Source: CAD feature listing. Evaluate the final solid. Frame: model axes, mm. Coordinates: 2 decimals unless noted, no trailing zeros. Order: outer loops, then holes, each group sorted by start corner. A loop starts at its lowest first (then second) coordinate and runs counter-clockwise, first axis right, second up.
Autodesk Inventor part; units mm, degrees
ref_plane "YZ Plane" through (0, 0, 0) normal (1, 0, 0) x (0, 1, 0)
ref_plane "XZ Plane" through (0, 0, 0) normal (0, 1, 0) x (-1, 0, 0)
ref_plane "XY Plane" through (0, 0, 0) normal (0, 0, 1) x (1, 0, 0)
sketch "Sketch1" plane through (0, 0, 0) normal (0, 0, 1) x (1, 0, 0)
  line L0 (0, 0) -> (127, 0)
  line L1 (127, 0) -> (127, 88.9)
  line L2 (127, 88.9) -> (0, 88.9)
  line L3 (0, 88.9) -> (0, 0)
  circle A0 centre (10.16, 78.74) radius 3.0988
  circle A1 centre (10.16, 44.45) radius 3.0988
  circle A2 centre (10.16, 10.16) radius 3.0988
  circle A3 centre (45.72, 10.16) radius 3.0988
  circle A4 centre (116.84, 10.16) radius 3.0988
  circle A5 centre (116.84, 44.45) radius 3.0988
  circle A6 centre (116.84, 78.74) radius 3.0988
  circle A7 centre (45.72, 78.74) radius 3.0988
  line L4 (25.4, 25.4) -> (101.6, 25.4)
  line L5 (101.6, 25.4) -> (101.6, 63.5)
  line L6 (101.6, 63.5) -> (25.4, 63.5)
  line L7 (25.4, 63.5) -> (25.4, 25.4)
  line L8 (25.4, 25.4) -> (101.6, 63.5) construction
  line L9 (101.6, 25.4) -> (25.4, 63.5) construction
  circle A8 centre (81.28, 10.16) radius 3.0988
  circle A9 centre (81.28, 78.74) radius 3.0988
  point P0 (63.5, 44.45)
  dimension "d0" = 127
  dimension "d1" = 88.9
  dimension "d3" = 6.1976
  dimension "d4" = 10.16
  dimension "d5" = 10.16
  dimension "d6" = 10.16
  dimension "d7" = 10.16
  dimension "d8" = 44.45
  dimension "d10" = 10.16
  dimension "d11" = 10.16
  dimension "d12" = 10.16
  dimension "d13" = 10.16
  dimension "d14" = 44.45
  dimension "d15" = 10.16
  dimension "d16" = 10.16
  dimension "d17" = 10.16
  dimension "d18" = 10.16
  dimension "d31" = 76.2
  dimension "d32" = 38.1
  dimension "d33" = 44.45
  dimension "d34" = 63.5
  dimension "d42" = 35.56
  dimension "d43" = 35.56
  dimension "d44" = 35.56
  dimension "d46" = 35.56
  dimension "d47" = 35.56
  dimension "d49" = 35.56
extrude "Extrusion1" add sketch "Sketch1" along normal blind 4.7625
thread "Thread1"
thread "Thread2"
thread "Thread3"
thread "Thread4"
thread "Thread5"
thread "Thread6"
thread "Thread7"
thread "Thread8"
thread "Thread9"
fillet "Fillet3" radius 12.7 4 edges at (101.6, 63.5, 2.3813) (101.6, 25.4, 2.3813) (25.4, 63.5, 2.3813) (25.4, 25.4, 2.3813)
sketch "Sketch4" plane through (0, 0, 4.7625) normal (0, 0, 1) x (1, 0, 0)
  arc A0 (38.1, 63.5) -> (25.4, 50.8) centre (38.1, 50.8) ccw
  arc A1 (38.1, 63.5) -> (25.4, 50.8) centre (38.1, 50.8) ccw
  arc A2 (101.6, 50.8) -> (88.9, 63.5) centre (88.9, 50.8) ccw
  arc A3 (101.6, 50.8) -> (88.9, 63.5) centre (88.9, 50.8) ccw
  arc A4 (88.9, 25.4) -> (101.6, 38.1) centre (88.9, 38.1) ccw
  arc A5 (88.9, 25.4) -> (101.6, 38.1) centre (88.9, 38.1) ccw
  arc A6 (25.4, 38.1) -> (38.1, 25.4) centre (38.1, 38.1) ccw
  arc A7 (25.4, 38.1) -> (38.1, 25.4) centre (38.1, 38.1) ccw
  line L0 (38.1, 25.4) -> (88.9, 25.4)
  line L1 (38.1, 25.4) -> (88.9, 25.4)
  line L2 (101.6, 38.1) -> (101.6, 50.8)
  line L3 (101.6, 38.1) -> (101.6, 50.8)
  line L4 (88.9, 63.5) -> (38.1, 63.5)
  line L5 (88.9, 63.5) -> (38.1, 63.5)
  line L6 (25.4, 38.1) -> (25.4, 50.8)
  line L7 (25.4, 50.8) -> (25.4, 38.1)
  arc A8 (38.1, 66.04) -> (22.86, 50.8) centre (38.1, 50.8) ccw
  line L8 (22.86, 50.8) -> (22.86, 38.1)
  arc A9 (22.86, 38.1) -> (38.1, 22.86) centre (38.1, 38.1) ccw
  line L9 (38.1, 22.86) -> (88.9, 22.86)
  arc A10 (88.9, 22.86) -> (104.14, 38.1) centre (88.9, 38.1) ccw
  line L10 (104.14, 38.1) -> (104.14, 50.8)
  arc A11 (104.14, 50.8) -> (88.9, 66.04) centre (88.9, 50.8) ccw
  line L11 (88.9, 66.04) -> (38.1, 66.04)
  arc A12 (38.1, 69.5198) -> (19.3802, 50.8) centre (38.1, 50.8) ccw
  line L12 (19.3802, 50.8) -> (19.3802, 38.1)
  arc A13 (19.3802, 38.1) -> (38.1, 19.3802) centre (38.1, 38.1) ccw
  line L13 (38.1, 19.3802) -> (88.9, 19.3802)
  arc A14 (88.9, 19.3802) -> (107.6198, 38.1) centre (88.9, 38.1) ccw
  line L14 (107.6198, 38.1) -> (107.6198, 50.8)
  arc A15 (107.6198, 50.8) -> (88.9, 69.5198) centre (88.9, 50.8) ccw
  line L15 (88.9, 69.5198) -> (38.1, 69.5198)
  point P0 (0, 0)
  dimension "d69" = 2.54
  dimension "d70" = 3.4798
extrude "Extrusion4" cut sketch "Sketch4" against normal blind 1.9812 contours L15 A15 L14 A14 L13 A13 L12 A12
thread "Thread10"
equation "\"d6\" = d5"
equation "\"d7\" = d4"
equation "\"d8\" = 0.5 * d1"
equation "\"d10\" = d4"
equation "\"d11\" = d5"
equation "\"d12\" = d4"
equation "\"d13\" = d5"
equation "\"d14\" = 0.5 * d1"
equation "\"d15\" = d13"
equation "\"d16\" = d12"
equation "\"d17\" = d13"
equation "\"d18\" = d16"
equation "\"d43\" = d42"
equation "\"d44\" = d43"
equation "\"d46\" = d42"
equation "\"d47\" = d46"
equation "\"d49\" = d46"
properties part number "Front"
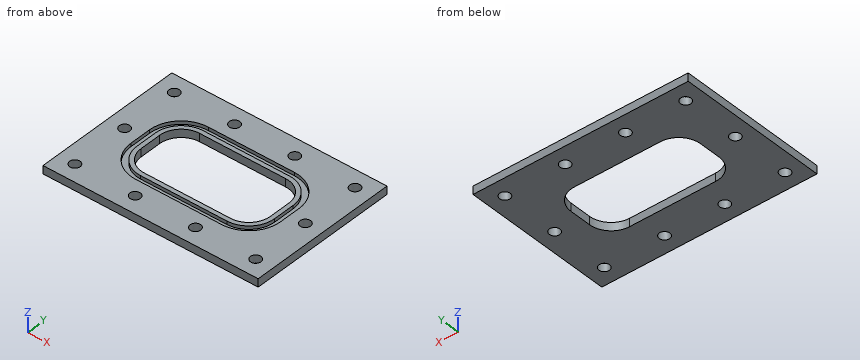
1. Pin query (flat end, axial travel): P1, Ø5, axis at x = 116.84, y = 78.74, coming from the -Z side. Return the tip coordinate at first contact, or that it passes through.
Findings:
P1: passes through
2. Section query B-B on z = 1.2. Count the separate pieces of the cut face and the enclosed holes in it, plus the area to 3 significant figures.
Findings:
separate pieces: 1
enclosed holes: 11
area: 8,220 mm2
3. Section query C-C on y = 78.74. Return loops of the section in (x, z), plus the area to 3 significant figures.
Findings:
outline: (0, 0) - (7.06, 0) - (7.06, 4.76) - (0, 4.76) - close; (13.26, 0) - (42.62, 0) - (42.62, 4.76) - (13.26, 4.76) - close; (48.82, 0) - (78.18, 0) - (78.18, 4.76) - (48.82, 4.76) - close; (84.38, 0) - (113.74, 0) - (113.74, 4.76) - (84.38, 4.76) - close; (119.94, 0) - (127, 0) - (127, 4.76) - (119.94, 4.76) - close
area: 487 mm2
4. Section query D-D on x = 116.84. Return loops of the section in (y, z), plus the area to 3 significant figures.
Findings:
outline: (0, 0) - (7.06, 0) - (7.06, 4.76) - (0, 4.76) - close; (13.26, 0) - (41.35, 0) - (41.35, 4.76) - (13.26, 4.76) - close; (47.55, 0) - (75.64, 0) - (75.64, 4.76) - (47.55, 4.76) - close; (81.84, 0) - (88.9, 0) - (88.9, 4.76) - (81.84, 4.76) - close
area: 335 mm2
5. Ray query, line 1 (Y direction, x = 78, z = 3.7); line 2 (Y direction, x = 10.16, z = 1.35); line 3 (X direction, y = 40, z = 4.05). Return the intervals inside material, ascending.
Findings:
line 1: y = 0 to 19.38, 22.86 to 25.4, 63.5 to 66.04, 69.52 to 88.9
line 2: y = 0 to 7.06, 13.26 to 41.35, 47.55 to 75.64, 81.84 to 88.9
line 3: x = 0 to 19.38, 22.86 to 25.4, 101.6 to 104.14, 107.62 to 127
6. Section query A-A on y = 44.45. Return loops of the section in (x, z).
Findings:
outline: (0, 0) - (7.06, 0) - (7.06, 4.76) - (0, 4.76) - close; (13.26, 0) - (25.4, 0) - (25.4, 4.76) - (22.86, 4.76) - (22.86, 2.78) - (19.38, 2.78) - (19.38, 4.76) - (13.26, 4.76) - close; (101.6, 0) - (113.74, 0) - (113.74, 4.76) - (107.62, 4.76) - (107.62, 2.78) - (104.14, 2.78) - (104.14, 4.76) - (101.6, 4.76) - close; (119.94, 0) - (127, 0) - (127, 4.76) - (119.94, 4.76) - close
